Design review of the part built by this model. Coordinates are the model's own, in mm. A direction names the side the tool comes from. Coordinates: 2 decimals unless noted, no trailing zeros. Loops run counter-clockwise (first coordinate to the right, second up) from the corner with the lowest first, then second, coordinate; pieces in that order, holes last.
Q1. Add section B-B on z = 31. Give the boundary of the cut face in (x, y), and give its area (3 significant figures).
Q2. Draft analysis for pull direction Y (two halves, no side actions). For faces 6 (the face through (-1.432, 56.906, 0.986)), 7 (the face through (0, -31, 43.5)), 8 (the face through (0, -4, -2)), state which applies: released by +Y, released by -Y, zero draft, split by the parting line, or undercut.
Q3. Add section C-C on x = -5. Give the number of separate pieces and of enclosed holes in the cut face, and give its area (3 significant figures).
Q4. Add section A-A on y = -56. Give the boundary of the cut face in (x, z).
Q5. Add section D-D on y = -21.5. Give the boundary of the cut face in (x, z).
Q6. Machinability: for faces 1 (the face through (0, 28, 0)), 2 (the face through (0, 74, 20)), 3 (the face through (0, -34, 41.5)), 4 (the face through (0, 28, 40)), 5 (the face through (0, 76, 20)), which of the approach directions +Z, -Z, +X, -X, +Y, -Y give a long, thin tool a straight path to every point of the face, cutting with its end or side? Answer none if there is none.
Q7. For P1, Ø8, axis at x = -2, y = 19, coming from the +Z side; P2, Ø4, axis at x = -6, z = 42.5, coming from the +Y side; P3, Ø1, axis at x = -3.5, z = 32.5, coming from the -Y side, all flat-tipped, find the tip position at first contact; note any pin that passes through.
Q8. Wall thickness on probe 1 along Z at (x, y) = (-11, -28); probe 2 along Y at (x, z) = (0, 42.05); probe 3 along Z at (x, y) = (3, 33): over which ranges is each line inside the solid? List them lowest first.
```python
from build123d import *

# Parameters (mm, degrees)
SKETCH1_W           = 28
SKETCH1_H           = 80
SKETCH1_R           = 11
BOSS_EXTRUDE1_DEPTH = 40
SKETCH1_4_W         = 28
SKETCH1_4_H         = 72
SKETCH1_4_R         = 13
BOSS_EXTRUDE2_DEPTH = 43.5
BOSS_EXTRUDE3_START = -3.5
SKETCH1_5_W         = 28
SKETCH1_5_H         = 72
SKETCH1_5_R         = 13
BOSS_EXTRUDE3_DEPTH = 3.5
SKETCH3_W           = 18
SKETCH3_H           = 76
CUT_EXTRUDE1_DEPTH  = 28
SKETCH3_4_W         = 21.5
SKETCH3_4_H         = 70
CUT_EXTRUDE2_DEPTH  = 28


with BuildPart() as part:
    # Sketch1 → Boss-Extrude1 (new body)
    with BuildSketch(Plane.XY):
        with Locations((0, 36)):
            Rectangle(SKETCH1_W, SKETCH1_H)
        with Locations((0, 46)):
            Circle(SKETCH1_R, mode=Mode.SUBTRACT)
    extrude(amount=BOSS_EXTRUDE1_DEPTH)

    # Sketch1_4 → Boss-Extrude2 (add)
    with BuildSketch(Plane.XY):
        with Locations((0, -40)):
            Rectangle(SKETCH1_4_W, SKETCH1_4_H)
        with Locations((0, -56)):
            Circle(SKETCH1_4_R, mode=Mode.SUBTRACT)
    extrude(amount=BOSS_EXTRUDE2_DEPTH)

    # Sketch1_5 → Boss-Extrude3 (add)
    with BuildSketch(Plane.XY.offset(BOSS_EXTRUDE3_START)):
        with Locations((0, -40)):
            Rectangle(SKETCH1_5_W, SKETCH1_5_H)
        with Locations((0, -56)):
            Circle(SKETCH1_5_R, mode=Mode.SUBTRACT)
    extrude(amount=BOSS_EXTRUDE3_DEPTH)

    # Sketch3 → Cut-Extrude1 (cut)
    with BuildSketch(Plane(origin=(14, 0, 0), x_dir=(0, 0, -1), z_dir=(1, 0, 0))):
        with Locations((-29, 36)):
            Rectangle(SKETCH3_W, SKETCH3_H)
        with Locations((-11, 36)):
            Rectangle(SKETCH3_W, SKETCH3_H)
    extrude(amount=-CUT_EXTRUDE1_DEPTH, mode=Mode.SUBTRACT)

    # Sketch3_4 → Cut-Extrude2 (cut)
    with BuildSketch(Plane(origin=(14, 0, 0), x_dir=(0, 0, -1), z_dir=(1, 0, 0))):
        with Locations((-9.25, -41)):
            Rectangle(SKETCH3_4_W, SKETCH3_4_H)
        with Locations((-30.75, -41)):
            Rectangle(SKETCH3_4_W, SKETCH3_4_H)
    extrude(amount=-CUT_EXTRUDE2_DEPTH, mode=Mode.SUBTRACT)


solid = part.part
```
Entries:
1. outline: (-14, -6) - (14, -6) - (14, -2) - (-14, -2) - close; (-14, 74) - (14, 74) - (14, 76) - (-14, 76) - close
1. area: 168 mm2
2. face 6: undercut
2. face 7: zero draft
2. face 8: released by +Y
3. separate pieces: 4
3. enclosed holes: 0
3. area: 664 mm2
4. outline: (-14, -3.5) - (-13, -3.5) - (-13, -1.5) - (-14, -1.5) - close; (-14, 41.5) - (-13, 41.5) - (-13, 43.5) - (-14, 43.5) - close; (13, -3.5) - (14, -3.5) - (14, -1.5) - (13, -1.5) - close; (13, 41.5) - (14, 41.5) - (14, 43.5) - (13, 43.5) - close
5. outline: (-14, -3.5) - (14, -3.5) - (14, -1.5) - (-14, -1.5) - close; (-14, 41.5) - (14, 41.5) - (14, 43.5) - (-14, 43.5) - close
6. face 1: -Z, +X, -X, +Y
6. face 2: +X, -X
6. face 3: +X, -X, -Y
6. face 4: +Z, +X, -X, +Y
6. face 5: +Z, -Z, +X, -X, +Y
7. P1: stops at z = 40
7. P2: stops at y = -4
7. P3: stops at y = -6
8. probe 1: z = -3.5 to -1.5, 41.5 to 43.5
8. probe 2: y = -76 to -69, -43 to -4
8. probe 3: z = 0 to 2, 38 to 40
